Source: three-view drawing plus pictorial views. Frame: mm from the lowest corner of the part. A direction names the side the tool comes from. Give positions to 0.01 mm unless a question says otherwise; leave off trailing zeros. Write each loop counter-clockwise with the first axis right and the second up, starting at its lowest first coordinate (ties: lowest second). Pieces come first, ordered by that corner, then holes. Notation, with made-up numbers: M 59,-35.5 L 97,-35.5 A6 ccw 97,-30.5 Z; hole C 88,53 d1. An arc over 180 degrees is marked long. Return JSON: item names as keys, results as strings.
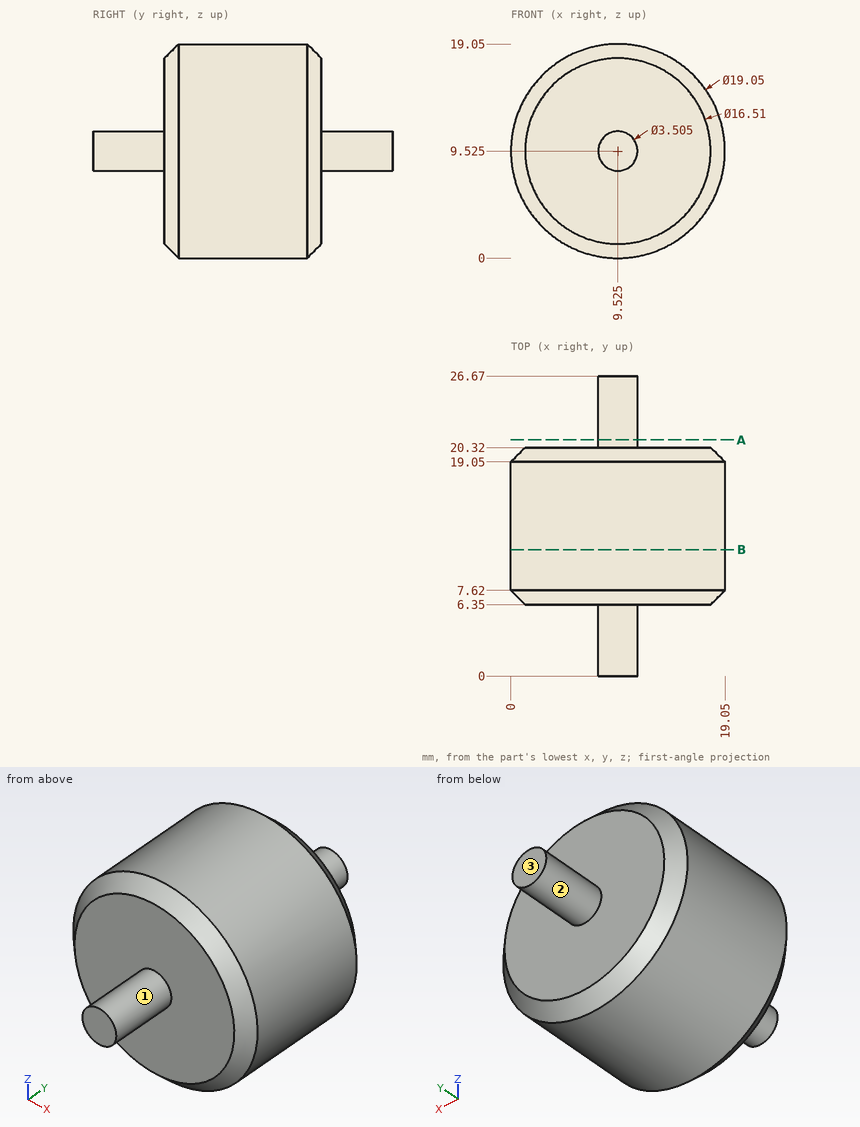
1) Set-up query: the marked faces 1, 2 and 3. Return all of +Z, -Z, +X, -X, +Y, -Y with unobstructed straight access to the full face (end or side cutting, diameter ignored); none if empty.
Numbers:
{"face 1": "-Y", "face 2": "+Y", "face 3": "+Z, -Z, +X, -X, +Y"}
2) Line query: line 1 (Y direction, x = 9.5, z = 2.75); line 2 (X direction, y = 19, z = 18); line 3 (Z direction, x = 9, y = 12). Output: solid intervals per line, ascending. Write a range as [from, to].
Numbers:
{"line 1": "y = [6.35, 20.32]", "line 2": "x = [5.18, 13.87]", "line 3": "z = [0.01, 19.04]"}
3) Contact query for flat-ended pins moving along their axis: pin 1 Ø1 at (x, z) = (7.5, 12) entering from +Y; pin 2 Ø4 at (y, z) = (7.5, 7) entering from -X; pin 3 Ø5 at (x, y) = (14.5, 20.5) entering from +Z (1 decimal). Output: stop coordinate, or through.
Numbers:
{"pin 1": "stops at y = 20.32", "pin 2": "stops at x = 0.01", "pin 3": "stops at z = 18.6"}
4) Cut plane A-A, the plane y = 21. Return the cut outline in (x, z) (1 decimal), then the cut area to 3 significant figures.
Numbers:
{"outline": "C 9.5,9.5 d3.5", "area": "9.65 mm²"}
5) Cut plane B-B, the plane y = 11.25. Return the cut outline in (x, z) (3 decimals).
Numbers:
{"outline": "C 9.525,9.525 d19.05"}
